For this review, take the finished solid that the model builds, in its own axes (mm). Give positions to 0.01 mm unless a question says otherwise; leave off trailing zeros. Order: outer loops, then holes, each group sorted by start corner. A loop starts at its lowest first (then second) coordinate and runs counter-clockwise, first axis right, second up.
Autodesk Inventor part; units mm, degrees
ref_plane "YZ Plane" through (0, 0, 0) normal (1, 0, 0) x (0, 1, 0)
ref_plane "XZ Plane" through (0, 0, 0) normal (0, 1, 0) x (-1, 0, 0)
ref_plane "XY Plane" through (0, 0, 0) normal (0, 0, 1) x (1, 0, 0)
sketch "Sketch1" plane through (0, 0, 0) normal (1, 0, 0) x (0, 1, 0)
  line L0 (-4.25, -58.4) -> (-75.9, -58.4)
  arc A0 (-78.2159, -55.4407) -> (-75.9, -58.4) centre (-75.9, -56.0141) ccw
  arc A1 (-78.2159, -55.4407) -> (-80.9407, -52.7159) centre (-80.4, -54.9) ccw
  arc A2 (-83.9, -50.4) -> (-80.9407, -52.7159) centre (-81.5141, -50.4) ccw
  line L1 (-83.9, -50.4) -> (-83.9, 50.4)
  arc A3 (-81.3323, 52.0522) -> (-83.9, 50.4) centre (-82.0846, 50.4) ccw
  arc A4 (-81.3323, 52.0522) -> (-78.2997, 54.9071) centre (-80.4, 54.1) ccw
  arc A5 (-75.9, 58.4) -> (-78.2997, 54.9071) centre (-75.9, 55.8292) ccw
  line L2 (-75.9, 58.4) -> (-4.25, 58.4)
  arc A6 (-2.25, 56.4) -> (-4.25, 58.4) centre (-4.25, 56.4) ccw
  line L3 (-2.25, 56.4) -> (-2.25, 54.5)
  arc A7 (-2.25, 54.5) -> (2.25, 54.5) centre (0, 54.5) ccw
  line L4 (2.25, 54.5) -> (2.25, 56.4)
  arc A8 (4.25, 58.4) -> (2.25, 56.4) centre (4.25, 56.4) ccw
  line L5 (4.25, 58.4) -> (75.9, 58.4)
  arc A9 (77.6729, 55.2614) -> (75.9, 58.4) centre (75.9, 56.33) ccw
  arc A10 (77.6729, 55.2614) -> (80.7614, 52.1729) centre (79.6, 54.1) ccw
  arc A11 (83.9, 50.4) -> (80.7614, 52.1729) centre (81.83, 50.4) ccw
  line L6 (83.9, 50.4) -> (83.9, -50.4)
  arc A12 (80.4071, -52.7997) -> (83.9, -50.4) centre (81.3292, -50.4) ccw
  arc A13 (80.4071, -52.7997) -> (77.5522, -55.8323) centre (79.6, -54.9) ccw
  arc A14 (75.9, -58.4) -> (77.5522, -55.8323) centre (75.9, -56.5846) ccw
  line L7 (75.9, -58.4) -> (4.25, -58.4)
  arc A15 (2.25, -56.4) -> (4.25, -58.4) centre (4.25, -56.4) ccw
  line L8 (2.25, -56.4) -> (2.25, -54.5)
  arc A16 (2.25, -54.5) -> (-2.25, -54.5) centre (0, -54.5) ccw
  line L9 (-2.25, -54.5) -> (-2.25, -56.4)
  arc A17 (-4.25, -58.4) -> (-2.25, -56.4) centre (-4.25, -56.4) ccw
  circle A18 centre (-80.4, -54.9) radius 1.25
  circle A19 centre (-80.4, 54.1) radius 1.25
  circle A20 centre (0, -54.5) radius 1.25
  circle A21 centre (79.6, -54.9) radius 1.25
  circle A22 centre (0, 54.5) radius 1.25
  circle A23 centre (79.6, 54.1) radius 1.25
  arc A24 (-85.9, -58.4) -> (-83.9, -60.4) centre (-83.9, -58.4) ccw
  line L10 (-83.9, -60.4) -> (83.9, -60.4)
  arc A25 (83.9, -60.4) -> (85.9, -58.4) centre (83.9, -58.4) ccw
  line L11 (85.9, -58.4) -> (85.9, 58.4)
  arc A26 (85.9, 58.4) -> (83.9, 60.4) centre (83.9, 58.4) ccw
  line L12 (83.9, 60.4) -> (-83.9, 60.4)
  arc A27 (-83.9, 60.4) -> (-85.9, 58.4) centre (-83.9, 58.4) ccw
  line L13 (-85.9, 58.4) -> (-85.9, -58.4)
  point P0 (0, 0)
  point P1 (0, 0)
extrude "Extrusion1" add sketch "Sketch1" along normal blind 2
properties part number "gasket"
1) Draft analysis for pull direction Y (two halves, no side actions). For faces 1 (the face through (0, 0, 58)), 2 (the face through (0.99, 78.04, 52.48)), state which applies: +Y half, -Y half, draft (parallel to the pull), parting line (faces both ways), or undercut.
Answer sheet:
face 1: draft
face 2: undercut
2) We need section A-A on y = -20.5. Give the boundary of the cut face in (x, z).
Answer sheet:
outline: (0, -60.4) - (2, -60.4) - (2, -58.4) - (0, -58.4) - close; (0, 58.4) - (2, 58.4) - (2, 60.4) - (0, 60.4) - close
3) We need section C-C on x = 0.85. Count the separate pieces of the cut face and the enclosed holes in it, then the cut area to 3 significant figures.
Answer sheet:
separate pieces: 1
enclosed holes: 7
area: 1,320 mm2
4) To check wall thickness, follow line 1 (Z direction, x = 1.1, y = 0); line 2 (Z direction, x = 0.5, y = -80.4); line 3 (Y direction, x = 0.4, z = 46). State the ranges of each line that lie inside material, in increasing order.
Answer sheet:
line 1: z = -60.4 to -55.75, -53.25 to -52.25, 52.25 to 53.25, 55.75 to 60.4
line 2: z = -60.4 to -56.15, -53.65 to -52.65, 51.85 to 52.85, 55.35 to 60.4
line 3: y = -85.9 to -83.9, 83.9 to 85.9
5) We need section B-B on z = -10. Give the boundary of the cut face in (x, y).
Answer sheet:
outline: (0, -85.9) - (2, -85.9) - (2, -83.9) - (0, -83.9) - close; (0, 83.9) - (2, 83.9) - (2, 85.9) - (0, 85.9) - close
6) Clearance check with a flat-ended pin moving along its axis: pin 1 (2 mm diameter, centred on y = 79.6, z = -54.9, fed in from -X). State where the tip first meets the part, or that it passes through.
Answer sheet:
pin 1: passes through
